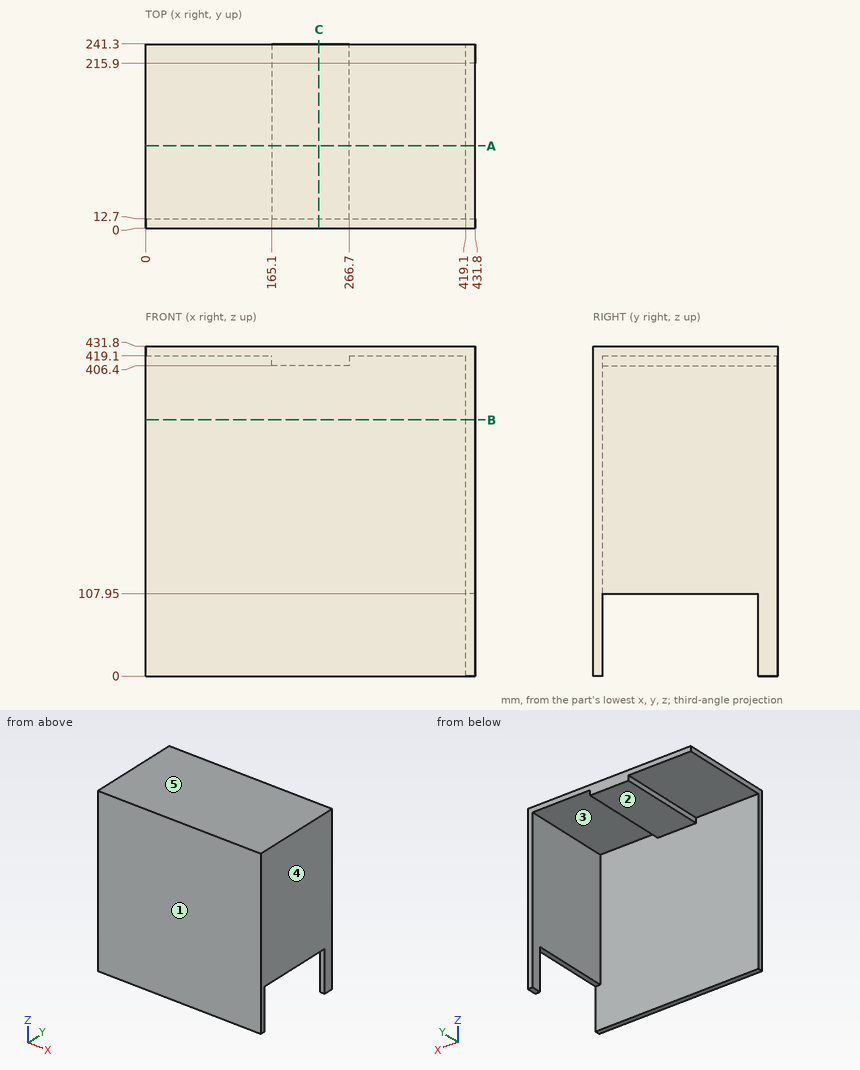
Job drawing, mm, ordinate dimensions from the low corner. One solid piece. A direction names the side the tool comes from. Coordinates: 2 decimals unless noted, no trailing zeros. Order: outer loops, then holes, each group sorted by start corner. A loop starts at its lowest first (then second) coordinate and runs counter-clockwise, first axis right, second up. Notation, with made-up numbers: (1.5, 21.5) -> (29.5, 21.5) arc R16 cw to (29.5, 37.5) -> close; hole circle Ø5 at (73.25, 43). An arc over 180 degrees is marked (long way). Put each result on its own line as item: value. Start each with the question number.
(1) Band-saw the part on A-A (y = 108). Give the cut face in (x, z).
(2) Band-saw the part on B-B (z = 335.5). Give the cut face in (x, y), then the cut area to 3 significant figures.
(3) Which spindle directions (+Z, -Z, +X, -X, +Y, -Y) get a long thin tool onto all of the face, cutting with end or side? Do the marked faces 1 and 2. Say none if no direction does.
(4) Mould opens along X. For the marked faces 3, 4 and 5 say: pulls with the +X half, pulls with the -X half, needs draft (parallel to the pull), parting line crosses it, or undercut.
(5) Pin check, flat tips, straight feed: pin 1 Ø4 at (x, y) = (422.5, 83.5) entering from -Z; pin 2 Ø6 at (x, y) = (166.5, 215.5) entering from -Z; pin 3 Ø6 at (x, z) = (144.5, 380.5) entering from +Y. Stop position of each tip, or through.
(6) Probe line 1 along X through (y, z) = (15.5, 129.5); line 2 along Y through (x, z) = (110.5, 109.5). List the from-to ranges inside material, lowest first. Write a range as [from, to].
(7) Band-saw the part on C-C (x = 227). Give the cut face in (y, z).
Determined:
1. outline: (0, 419.1) -> (165.1, 419.1) -> (165.1, 406.4) -> (266.7, 406.4) -> (266.7, 419.1) -> (419.1, 419.1) -> (419.1, 107.95) -> (431.8, 107.95) -> (431.8, 431.8) -> (0, 431.8) -> close
2. outline: (0, 0) -> (431.8, 0) -> (431.8, 241.3) -> (419.1, 241.3) -> (419.1, 12.7) -> (0, 12.7) -> close
2. area: 8,390 mm²
3. face 1: +Z, -Z, +X, -X, -Y
3. face 2: -Z, -X, +Y
4. face 3: undercut
4. face 4: pulls with the +X half
4. face 5: needs draft
5. pin 1: stops at z = 107.95
5. pin 2: stops at z = 406.4
5. pin 3: stops at y = 12.7
6. line 1: x = [419.1, 431.8]
6. line 2: y = [0, 12.7]
7. outline: (0, 0) -> (12.7, 0) -> (12.7, 406.4) -> (241.3, 406.4) -> (241.3, 431.8) -> (0, 431.8) -> close
